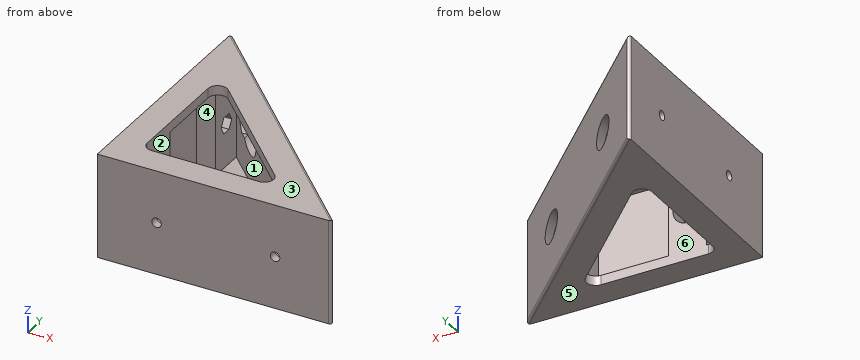
from build123d import *

# Parameters (mm, degrees)
PAD003_DEPTH    = 44
POCKET007_DEPTH = 36
SKETCH025_W     = 12
SKETCH025_H     = 16
SKETCH025_W_2   = 16
SKETCH025_H_2   = 12
PAD004_DEPTH    = 44
SKETCH026_R     = 2
POCKET008_DEPTH = 100
SKETCH027_R     = 6
POCKET009_DEPTH = 100
SKETCH028_R     = 2
POCKET010_DEPTH = 100
POCKET011_DEPTH = 100
FILLET007_R     = 1


with BuildPart() as part:
    # Sketch023 → Pad003 (new body)
    with BuildSketch(Plane.XY):
        Polygon((0, 100), (0, 0), (100, 0), align=None)
        with BuildLine():
            Line((12, 16), (12, 61.372583))
            ThreePointArc((18.828427, 64.20101), (14.469266, 65.068101), (12, 61.372583))
            Line((18.828427, 64.20101), (64.20101, 18.828427))
            ThreePointArc((61.372583, 12), (65.068101, 14.469266), (64.20101, 18.828427))
            Line((16, 12), (61.372583, 12))
            ThreePointArc((12, 16), (13.171573, 13.171573), (16, 12))
        make_face(mode=Mode.SUBTRACT)
    extrude(amount=PAD003_DEPTH)

    # Sketch024 → Pocket007 (cut)
    with BuildSketch(Plane(origin=(-1, 0, 4), x_dir=(1, 0, 0), z_dir=(0, 0, 1))):
        with BuildLine():
            Line((5, 80.686292), (5, 8))
            ThreePointArc((5, 8), (6.171573, 5.171573), (9, 4))
            Line((9, 4), (81.686292, 4))
            ThreePointArc((81.686292, 4), (85.38181, 6.469266), (84.514719, 10.828427))
            Line((84.514719, 10.828427), (11.828427, 83.514719))
            ThreePointArc((11.828427, 83.514719), (7.469266, 84.38181), (5, 80.686292))
        make_face()
    extrude(amount=POCKET007_DEPTH, mode=Mode.SUBTRACT)

    # Sketch025 → Pad004 (join)
    with BuildSketch(Plane.XY):
        with Locations((6, 75)):
            Rectangle(SKETCH025_W, SKETCH025_H)
        with Locations((6, 25)):
            Rectangle(SKETCH025_W, SKETCH025_H)
        with Locations((25, 6)):
            Rectangle(SKETCH025_W_2, SKETCH025_H_2)
        with Locations((75, 6)):
            Rectangle(SKETCH025_W_2, SKETCH025_H_2)
    extrude(amount=PAD004_DEPTH)

    # Sketch026 → Pocket008 (cut)
    with BuildSketch(Plane.XZ):
        with Locations((25, 22)):
            Circle(SKETCH026_R)
        with Locations((75, 22)):
            Circle(SKETCH026_R)
    extrude(amount=-POCKET008_DEPTH, mode=Mode.SUBTRACT)

    # Sketch027 → Pocket009 (cut)
    with BuildSketch(Plane.XZ.offset(-3.529412)):
        with Locations((25, 22)):
            Circle(SKETCH027_R)
        with Locations((75, 22)):
            Circle(SKETCH027_R)
    extrude(amount=-POCKET009_DEPTH, mode=Mode.SUBTRACT)

    # Sketch028 → Pocket010 (cut)
    with BuildSketch(Plane.YZ):
        with Locations((75, 22)):
            Circle(SKETCH028_R)
        with Locations((25, 22)):
            Circle(SKETCH028_R)
    extrude(amount=POCKET010_DEPTH, mode=Mode.SUBTRACT)

    # Sketch029 → Pocket011 (cut)
    with BuildSketch(Plane.YZ.offset(3.529412)):
        Polygon((21.05, 21.999978), (23.025, 18.579178), (26.975, 18.579178), (28.95, 21.999978), (26.975, 25.420778), (23.025, 25.420778), align=None)
        Polygon((76.975, 25.4208), (73.025, 25.4208), (71.05, 22), (73.025, 18.5792), (76.975, 18.5792), (78.95, 22), align=None)
    extrude(amount=POCKET011_DEPTH, mode=Mode.SUBTRACT)

    # Fillet007
    fillet007_edges = [part.edges().sort_by_distance(p)[0] for p in [
        (50, 50, 44),
        (50, 50, 0),
        (100, 0, 22),
        (0, 100, 22),
    ]]
    fillet(fillet007_edges, radius=FILLET007_R)


solid = part.part
For this review, take the finished solid that the model builds, in its own axes (mm). Face numbers are marked on the shaded views. A direction names the side the tool comes from. Give positions to 0.01 mm unless a question says otherwise; leave off trailing zeros. Answer as a JSON object with one key per item and string values. Group by question number.
Item 1: Clearance check with flat-ended pins moving along their axes: pin 1 Ø13 at (x, z) = (25, 25) entering from +Y; pin 2 Ø4 at (y, z) = (7, 19.5) entering from +X; pin 3 Ø10 at (y, z) = (11.5, 17) entering from +X; pin 4 Ø7 at (x, z) = (25, 22) entering from -Y. State where each tip first meets the part, or that it passes through.
Item 2: Machinability: for the marked faces 1, 2 and 3, which of the approach directions +Z, -Z, +X, -X, +Y, -Y give a long, thin tool a straight path to every point of the face, cutting with its end or side? Answer none if there is none.
Item 3: Take a section at A-A on x = 25. Give the number of separate pieces and of enclosed holes in the cut face, and give its area (3 significant figures).
Item 4: Wall thickness on line 1 along Y through (x, z) = (1.05, 22); line 2 along Z through (x, y) = (42, 50.5); line 3 along Y through (x, z) = (81, 39.5): over which ranges is each line inside the solid? List them lowest first.
Item 5: Draft analysis for pull direction Z (two halves, no side actions). For the marked faces 4, 5 and 6, state which applies: pulls with the +Z half, pulls with the -Z half, needs draft (parallel to the pull), parting line crosses it, or undercut.
Reported:
{
 "1": {"pin 1": "y = 81.5", "pin 2": "x = 95", "pin 3": "x = 93.5", "pin 4": "y = 0"},
 "2": {"face 1": "none", "face 2": "+Z, -Z", "face 3": "+Z, +X, -X, +Y, -Y"},
 "3": {"separate pieces": "4", "enclosed holes": "0", "area": "683 mm^2"},
 "4": {"line 1": "0 to 23, 27 to 73, 77 to 98.58", "line 2": "0 to 4, 40 to 44", "line 3": "0 to 12, 13.34 to 19"},
 "5": {"face 4": "undercut", "face 5": "pulls with the -Z half", "face 6": "needs draft"}
}
